```python
from build123d import *

# Parameters (mm, degrees)
SKETCH1_W               = 38.608
SKETCH1_H               = 38.608
BOSS_EXTRUDE1_DEPTH     = 19.304
CUT_EXTRUDE1_DEPTH      = 34.435508789
CUT_EXTRUDE1_DEPTH_BACK = 34.435508789
SKETCH2_R               = 12.7
CUT_EXTRUDE3_DEPTH      = 48.284949995
CUT_EXTRUDE3_DEPTH_BACK = 48.284949995
SKETCH3_R               = 12.7
CUT_EXTRUDE4_DEPTH      = 17.526
CUT_EXTRUDE5_DEPTH      = 34.435508789


with BuildPart() as part:
    # Sketch1 → Boss-Extrude1 (new, symmetric)
    with BuildSketch(Plane(origin=(0, 0, 0), x_dir=(1, 0, 0), z_dir=(0, 1, 0))):
        Rectangle(SKETCH1_W, SKETCH1_H)
    extrude(amount=BOSS_EXTRUDE1_DEPTH, both=True)

    # Sketch2 → Cut-Extrude1 (cut, two sides: drawn at the far end of the back side and taken through both)
    with BuildSketch(Plane.XY.offset(-CUT_EXTRUDE1_DEPTH_BACK)):
        Circle(SKETCH2_R)
    extrude(amount=CUT_EXTRUDE1_DEPTH + CUT_EXTRUDE1_DEPTH_BACK, mode=Mode.SUBTRACT)

    # Sketch3 → Cut-Extrude3 (cut, two sides: drawn at the far end of the back side and taken through both)
    with BuildSketch(Plane(origin=(0, 19.304, 0), x_dir=(0, 0, -1), z_dir=(0, -1, 0)).offset(-CUT_EXTRUDE3_DEPTH_BACK)):
        Circle(SKETCH3_R)
    extrude(amount=CUT_EXTRUDE3_DEPTH + CUT_EXTRUDE3_DEPTH_BACK, mode=Mode.SUBTRACT)

    # Sketch4 → Cut-Extrude4 (cut, symmetric)
    with BuildSketch(Plane(origin=(0, 0, 0), x_dir=(0, 0, -1), z_dir=(1, 0, 0))):
        Polygon((-17.376795594, -19.621859625), (19.621859625, 17.376795594), (17.376795594, 19.621859625), (-19.621859625, -17.376795594), align=None)
    extrude(amount=CUT_EXTRUDE4_DEPTH, both=True, mode=Mode.SUBTRACT)

    # Sketch4<2> → Cut-Extrude5 (cut, through all)
    with BuildSketch(Plane(origin=(0, 0, 0), x_dir=(0, 0, -1), z_dir=(1, 0, 0))):
        Polygon((-17.376795594, -19.621859625), (19.621859625, 17.376795594), (17.376795594, 19.621859625), (-19.621859625, -17.376795594), align=None)
    extrude(amount=CUT_EXTRUDE5_DEPTH, mode=Mode.SUBTRACT)


solid = part.part
```
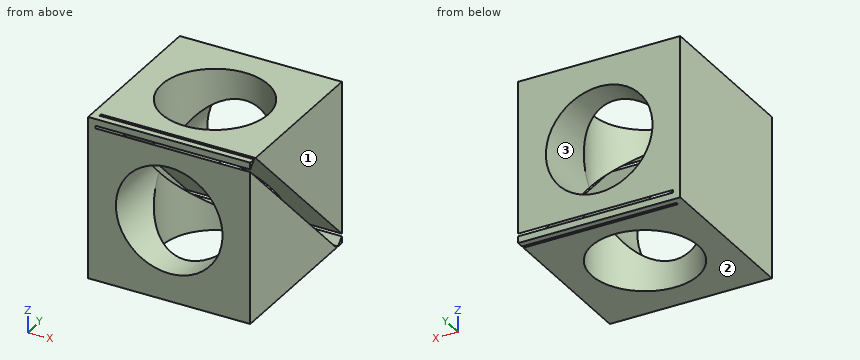
Verification items for the finished model (mm, model axes). Face numbers are marked on the shaded views. Coordinates: 2 decimals unless noted, no trailing zeros. Order: outer loops, then holes, each group sorted by start corner. A loop starts at its lowest first (then second) coordinate and runs counter-clockwise, first axis right, second up. Notation, with made-up numbers: (-17.5, 10) -> (37.5, 10) arc R28 ccw to (37.5, 43) -> close; hole circle Ø8 at (54.5, -14). An arc over 180 degrees is marked (long way). Put each result on its own line as item: value. Start each with the question number.
1) Material ranges on L1, parallel to X at y = 0, z = 8; L2, parallel to Z at x = 10.5, y = -16; L3, parallel to Y at x = -14.5, z = 13.5, recorded low to high.
2) Cross-section at B-B (y = 0). Enter the section's corners in (x, z), plus the area to 3 significant figures.
3) Go/stop test with flat-tipped pins: pin 1 (3 mm diameter, centred on x = 9, y = 2, fed in from +Z); pin 2 (2 mm diameter, centred on y = -3, z = 4, fed in from +X). Record where each tip stops, or that it passes through.
4) Cross-section at A-A (x = 15). Enter the section's corners in (y, z).
5) Release check for a two-part mould opening along X. For the marked faces 1, 2 and 3 record: pulls with the +X half, pulls with the -X half, needs draft (parallel to the pull), parting line crosses it, or undercut.
6) Cross-section at C-C (x = 0). Enter the section's corners in (y, z).
Geometry check:
1. L1: x = -19.3 to -12.7, 12.7 to 19.3
1. L2: z = -19.3 to -7.14, 7.14 to 13.75, 18.25 to 19.3
1. L3: y = -19.3 to -15.75, -11.25 to 19.3
2. outline: (-19.3, -19.3) -> (-12.7, -19.3) -> (-12.7, -2.25) -> (-17.53, -2.25) -> (-17.53, 2.25) -> (-12.7, 2.25) -> (-12.7, 19.3) -> (-19.3, 19.3) -> close; (12.7, -19.3) -> (19.3, -19.3) -> (19.3, -2.25) -> (12.7, -2.25) -> close; (12.7, 2.25) -> (19.3, 2.25) -> (19.3, 19.3) -> (12.7, 19.3) -> close
2. area: 459 mm^2
3. pin 1: passes through
3. pin 2: stops at x = 19.3
4. outline: (-19.3, -19.3) -> (17.06, -19.3) -> (-19.3, 17.06) -> close; (-19.3, 17.69) -> (-17.69, 19.3) -> (-19.3, 19.3) -> close; (-17.06, 19.3) -> (19.3, -17.06) -> (19.3, 19.3) -> close; (17.69, -19.3) -> (19.3, -19.3) -> (19.3, -17.69) -> close
5. face 1: pulls with the +X half
5. face 2: needs draft
5. face 3: undercut
6. outline: (-19.3, -19.3) -> (-12.7, -19.3) -> (-12.7, -12.7) -> (-19.3, -12.7) -> close; (-19.3, 12.7) -> (-14.95, 12.7) -> (-19.3, 17.06) -> close; (-19.3, 17.69) -> (-17.69, 19.3) -> (-19.3, 19.3) -> close; (-17.06, 19.3) -> (-12.7, 14.95) -> (-12.7, 19.3) -> close; (12.7, -19.3) -> (17.06, -19.3) -> (12.7, -14.95) -> close; (12.7, 12.7) -> (19.3, 12.7) -> (19.3, 19.3) -> (12.7, 19.3) -> close; (14.95, -12.7) -> (19.3, -17.06) -> (19.3, -12.7) -> close; (17.69, -19.3) -> (19.3, -19.3) -> (19.3, -17.69) -> close
